Check sheet for the modelled part. Datum: model origin and axes. Units: mm. Face numbers are marked on the shaded views. A direction names the side the tool comes from. Round coordinates to 2 decimals unless told otherwise and drop trailing zeros. Order: outer loops, then holes, each group sorted by start corner. A loop starts at its lowest first (then second) coordinate and runs counter-clockwise, first axis right, second up. Notation, with made-up numbers: (-16.5, 7) -> (39.5, 7) arc R26 cw to (39.5, 32) -> close; hole circle Ø3 at (-4, -30.75). An arc over 180 degrees is marked (long way). Answer in a Markdown table with one row per item. Add a question column.
1. Draft check along Y on the marked faces 3, 4 and 5. Enter one of: +Y half, -Y half, draft (parallel to the pull), parting line (faces both ways), or undercut.
2. Sectioned sample at C-C, the plane z = 0.75. Record the boundary of the cut face in (x, y).
3. Access from +Z, -Z, +X, -X, +Y, -Y to the whole of each face (thin tool, end or side, straight path). Record for the marked faces 1 and 2.
4. Sectioned sample at A-A, the plane x = 0. Record the boundary of the cut face in (y, z).
5. Material ranges on L1, parallel to Y at x = 0, z = 0.6; L2, parallel to Y at x = 0, z = 2.8; L3, parallel to Z at x = 5, y = -3.75, recorded low to high. Write a range as from..to.
6. Sectioned sample at D-D, the plane x = 4.5. Record the boundary of the cut face in (y, z).
7. Depth check by flat-ended pin: P1, Ø5.5, axis at x = 0.5, y = 0.5, coming from the +Z side; P2, Ø9, axis at x = 0, y = 0, coming from the +Z side. Enter the tip coordinate at first touch or a pass-through.
```python
from build123d import *

# Parameters (mm, degrees)
F0_R     = 6
F0_R_2   = 5
F1_DEPTH = 4
F0_R_3   = 7.5
F2_DEPTH = 0.5
F0_R_4   = 3.5
F3_DEPTH = 1.9
F0_R_5   = 1.75
F4_DEPTH = 1


with BuildPart() as f1:
    # F0 (on Top) → F1 (new body)
    with BuildSketch(Plane.XY):
        Circle(F0_R)
        Circle(F0_R_2, mode=Mode.SUBTRACT)
    extrude(amount=F1_DEPTH)

    # F0 (on Top) → F2 (join)
    with BuildSketch(Plane.XY):
        Circle(F0_R_3)
        Circle(F0_R, mode=Mode.SUBTRACT)
    extrude(amount=F2_DEPTH)

    # F0 (on Top) → F3 (join, through all)
    with BuildSketch(Plane.XY):
        Circle(F0_R_2)
        Circle(F0_R_4, mode=Mode.SUBTRACT)
    extrude(amount=F3_DEPTH)

    # F0 (on Top) → F4 (join)
    with BuildSketch(Plane.XY):
        Circle(F0_R_4)
        Circle(F0_R_5, mode=Mode.SUBTRACT)
    extrude(amount=F4_DEPTH)


solid = f1.part
```
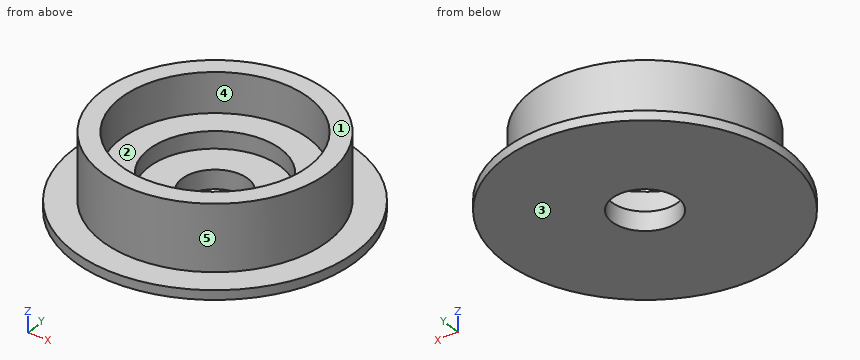
Answer key:
| question | item | result |
|---|---|---|
| 1 | face 3 | draft |
| 1 | face 4 | undercut |
| 1 | face 5 | parting line |
| 2 | outline | circle Ø12 at (0, 0); hole circle Ø3.5 at (0, 0) |
| 3 | face 1 | +Z, +X, -X, +Y, -Y |
| 3 | face 2 | +Z |
| 4 | outline | (-7.5, 0) -> (-1.75, 0) -> (-1.75, 1) -> (-3.5, 1) -> (-3.5, 1.9) -> (-5, 1.9) -> (-5, 4) -> (-6, 4) -> (-6, 0.5) -> (-7.5, 0.5) -> close; (1.75, 0) -> (7.5, 0) -> (7.5, 0.5) -> (6, 0.5) -> (6, 4) -> (5, 4) -> (5, 1.9) -> (3.5, 1.9) -> (3.5, 1) -> (1.75, 1) -> close |
| 5 | L1 | y = -6..-1.75, 1.75..6 |
| 5 | L2 | y = -6..-5, 5..6 |
| 5 | L3 | z = 0..0.5 |
| 6 | outline | (-6, 0) -> (6, 0) -> (6, 0.5) -> (3.97, 0.5) -> (3.97, 4) -> (2.18, 4) -> (2.18, 1.9) -> (-2.18, 1.9) -> (-2.18, 4) -> (-3.97, 4) -> (-3.97, 0.5) -> (-6, 0.5) -> close |
| 7 | P1 | stops at z = 1 |
| 7 | P2 | stops at z = 1.9 |
